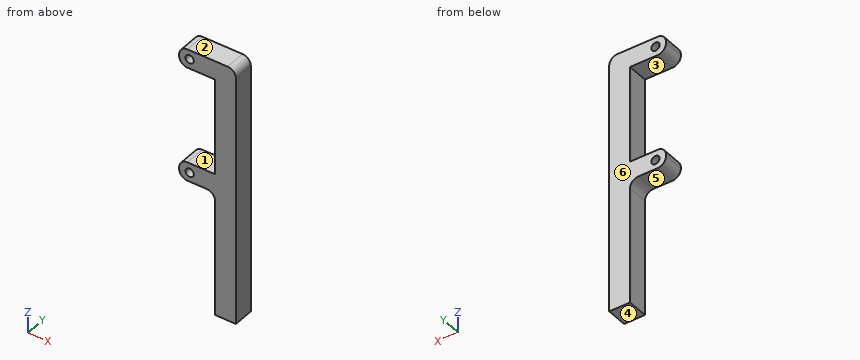
```python
from build123d import *

# Parameters (mm, degrees)
SKETCH1_R           = 1
BOSS_EXTRUDE1_DEPTH = 5
FILLET1_R           = 2


with BuildPart() as part:
    # Sketch1 → Boss-Extrude1 (new body)
    with BuildSketch(Plane(origin=(0, 0, 0), x_dir=(1, 0, 0), z_dir=(0, 1, 0))):
        Polygon((0, 4.5), (8.6, 4.5), (8.6, 27.7), (0, 27.7), (0, 32.2), (8.6, 32.2), (8.6, 62.2), (13.6, 62.2), (13.6, 0), (0, 0), align=None)
        with Locations(Location((2.5, 2.2, 0), (0, 0, 270))):
            Circle(SKETCH1_R, mode=Mode.SUBTRACT)
        with Locations(Location((2.5, 30, 0), (0, 0, 270))):
            Circle(SKETCH1_R, mode=Mode.SUBTRACT)
    extrude(amount=BOSS_EXTRUDE1_DEPTH)

    # Fillet1
    fillet1_edges = [part.edges().sort_by_distance(p)[0] for p in [
        (0, 2.5, -4.5),
        (0, 2.5, -27.7),
        (0, 2.5, -32.2),
        (8.6, 2.5, -32.2),
        (13.6, 2.5, 0),
        (0, 2.5, 0),
    ]]
    fillet(fillet1_edges, radius=FILLET1_R)


solid = part.part
```
Part model, mm, in its own coordinate system. Face numbers are marked on the shaded views. A direction names the side the tool comes from. Coordinates: 2 decimals unless noted, no trailing zeros. Order: outer loops, then holes, each group sorted by start corner. A loop starts at its lowest first (then second) coordinate and runs counter-clockwise, first axis right, second up. Notation, with made-up numbers: (28.25, 87.25) - (47.25, 87.25) arc R28 cw to (47.25, 120.25) - close; hole circle Ø11 at (5, 37.25). An arc over 180 degrees is marked (long way). Return JSON: item names as keys, results as strings. Group by question number.
Item 1: Which spindle directions (+Z, -Z, +X, -X, +Y, -Y) get a long thin tool onto all of the face, cutting with end or side? Do the marked faces 5 and 6. Say none if no direction does.
Item 2: Pull direction Z, two halves, no side cores. Call the marked faces 1, 2, 3 and 4: pulls with the +Z half, pulls with the -Z half, needs draft (parallel to the pull), parting line crosses it, or undercut.
Item 3: Cut at B-B (z = -50). List the corners of the cut face in (x, y), plus the area to 3 significant figures.
Item 4: Pin check, flat tips, straight feed: pin 1 (1 mm diameter, centred on x = 6.5, y = 1, fed in from -Z); pin 2 (2 mm diameter, centred on x = 6.5, y = 1.5, fed in from -Z); pin 3 (1.5 mm diameter, centred on y = 2, z = -16.5, fed in from -X). Stop position of each tip, or through.
Item 5: Drill centre lines: probe 1 along Z at (x, y) = (4.25, 1.2); probe 2 along X at (y, z) = (1.3, -2.2); probe 3 along X at (y, z) = (3.05, -19). Where is each one in solid material? Low to high. Write a range as from..to.
Item 6: Cut at A-A (y = 1.05). List the corners of the cut face in (x, z).
Check values:
{
 "1": {"face 5": "-Z, -X, +Y, -Y", "face 6": "+Z, -Z, +X, -X, +Y"},
 "2": {"face 1": "undercut", "face 2": "pulls with the +Z half", "face 3": "undercut", "face 4": "pulls with the -Z half"},
 "3": {"outline": "(8.6, 0) - (13.6, 0) - (13.6, 5) - (8.6, 5) - close", "area": "25.0 mm2"},
 "4": {"pin 1": "stops at z = -32.24", "pin 2": "stops at z = -32.41", "pin 3": "stops at x = 8.6"},
 "5": {"probe 1": "z = -32.2..-27.7, -4.5..0", "probe 2": "x = 0..1.5, 3.5..13.6", "probe 3": "x = 8.6..13.6"},
 "6": {"outline": "(0, -30.2) arc R2 ccw to (2, -32.2) - (6.6, -32.2) arc R2 cw to (8.6, -34.2) - (8.6, -62.2) - (13.6, -62.2) - (13.6, -2) arc R2 ccw to (11.6, 0) - (2, 0) arc R2 ccw to (0, -2) - (0, -2.5) arc R2 ccw to (2, -4.5) - (8.6, -4.5) - (8.6, -27.7) - (2, -27.7) arc R2 ccw to (0, -29.7) - close; hole circle Ø2 at (2.5, -30); hole circle Ø2 at (2.5, -2.2)"}
}
